Autodesk Inventor part; units mm, degrees
ref_plane "YZ Plane" through (0, 0, 0) normal (1, 0, 0) x (0, 1, 0)
ref_plane "XZ Plane" through (0, 0, 0) normal (0, 1, 0) x (-1, 0, 0)
ref_plane "XY Plane" through (0, 0, 0) normal (0, 0, 1) x (1, 0, 0)
sketch "Sketch1" plane through (0, 0, 0) normal (0, 0, 1) x (1, 0, 0)
  line L0 (-37.5, 37.5) -> (37.5, 37.5)
  line L1 (37.5, 37.5) -> (37.5, -37.5)
  line L2 (37.5, -37.5) -> (-37.5, -37.5)
  line L3 (-37.5, -37.5) -> (-37.5, 37.5)
  line L4 (-37.5, 37.5) -> (37.5, -37.5) construction
  line L5 (37.5, 37.5) -> (-37.5, -37.5) construction
  circle A0 centre (0, 0) radius 37.5
  circle A1 centre (19, -19) radius 2.4585
  circle A2 centre (19, 19) radius 2.4585
  circle A3 centre (-19, 19) radius 2.4585
  circle A4 centre (-19, -19) radius 2.4585
  point P0 (0, 0)
extrude "Extrusion1" add sketch "Sketch1" along normal blind 5
sketch "Sketch2" plane through (37.5, -37.5, 0) normal (1, 0, 0) x (0, 0, -1)
  line L0 (25.7498, -847.0546) -> (318.6402, 246.0273)
  line L1 (-5, 75) -> (-5, 0)
  line L2 (-5, 75) -> (272.8136, 75)
  line L3 (252.7174, 0) -> (-5, 0)
  point P0 (0, 37.5)
extrude "Extrusion2" add sketch "Sketch2" along normal blind 5
mirror "Mirror1" about plane through (0, 0, 0) normal (1, 0, 0) of "Extrusion2"
properties part number "Soporte Cilindro Cortadora"
Design review of the part built by this model. Coordinates are the model's own, in mm. A direction names the side the tool comes from. Coordinates: 2 decimals unless noted, no trailing zeros. Loops run counter-clockwise (first coordinate to the right, second up) from the corner with the lowest first, then second, coordinate; pieces in that order, holes last. Notation, with made-up numbers: (-12.5, 4.25) -> (-0.5, 4.25) arc R16 cw to (-0.5, 29.25) -> close; hole circle Ø3 at (35, 51). An arc over 180 degrees is marked (long way). Answer as a JSON object with one key per item and string values.
Q1. Clearance check with flat-ended pins moving along their axes: pin 1 Ø5 at (x, y) = (-13, -7) entering from -Z; pin 2 Ø5.5 at (x, y) = (-19, 19) entering from +Z. State where each tip first meets the part, or that it passes through.
Answer block:
{"pin 1": "stops at z = 0", "pin 2": "stops at z = 5"}
Q2. Take a section at D-D on x = -12. Give the boundary of the cut face in (y, z).
Answer block:
{"outline": "(-37.5, 0) -> (37.5, 0) -> (37.5, 5) -> (-37.5, 5) -> close"}
Q3. Take a section at B-B on z = -245. Give the boundary of the cut face in (x, y), plus the area to 3 significant figures.
Answer block:
{"outline": "(-42.5, -37.5) -> (-37.5, -37.5) -> (-37.5, 37.5) -> (-42.5, 37.5) -> close; (37.5, -37.5) -> (42.5, -37.5) -> (42.5, 37.5) -> (37.5, 37.5) -> close", "area": "750 mm^2"}
Q4. Take a section at C-C on y = -19. Give the boundary of the cut face in (x, z), plus the area to 3 significant figures.
Answer block:
{"outline": "(-42.5, -257.67) -> (-37.5, -257.67) -> (-37.5, 0) -> (-21.46, 0) -> (-21.46, 5) -> (-42.5, 5) -> close; (-16.54, 0) -> (16.54, 0) -> (16.54, 5) -> (-16.54, 5) -> close; (21.46, 0) -> (37.5, 0) -> (37.5, -257.67) -> (42.5, -257.67) -> (42.5, 5) -> (21.46, 5) -> close", "area": "2,950 mm^2"}
Q5. Tool access review of faces 5 (the flat face through (-42.5, 1, -136)), 6 (the flat face through (37.5, 1, -134)): name each direction out of +Z, -Z, +X, -X, +Y, -Y from which nothing blocks a thin tool from reaching the whole face with its end or side.
Answer block:
{"face 5": "+Z, -Z, -X, +Y, -Y", "face 6": "-Z, +Y, -Y"}
Q6. Take a section at A-A on x = 19. Give the boundary of the cut face in (y, z), plus the area to 3 significant figures.
Answer block:
{"outline": "(-37.5, 0) -> (-21.46, 0) -> (-21.46, 5) -> (-37.5, 5) -> close; (-16.54, 0) -> (16.54, 0) -> (16.54, 5) -> (-16.54, 5) -> close; (21.46, 0) -> (37.5, 0) -> (37.5, 5) -> (21.46, 5) -> close", "area": "326 mm^2"}
Q7. The part is to be moulded in two halves that separate along Y. For faces 1 (the cylindrical face through (-21.456, -19.108, 2.465)), 2 (the flat face through (-40, 0.5, -262.9)), 3 (the flat face through (38, 37.5, -135)), 4 (the cylindrical face through (16.544, -19.108, 2.465)), say which applies: +Y half, -Y half, draft (parallel to the pull), parting line (faces both ways), or undercut.
Answer block:
{"face 1": "undercut", "face 2": "-Y half", "face 3": "+Y half", "face 4": "undercut"}
Q8. To check wall thickness, follow L1, parallel to Y at x = -19, z = 1.65; L2, parallel to X at y = -22.5, z = -83; L3, parallel to Z at x = -14, y = 22. State the ranges of each line that lie inside material, in increasing order.
Answer block:
{"L1": "y = -37.5 to -21.46, -16.54 to 16.54, 21.46 to 37.5", "L2": "x = -42.5 to -37.5, 37.5 to 42.5", "L3": "z = 0 to 5"}
